CAD build for the part. Positions are in the model's coordinates, mm. Face numbers are marked on the shaded views. A direction names the side the tool comes from. Coordinates: 2 decimals unless noted, no trailing zeros. Loops run counter-clockwise (first coordinate to the right, second up) from the corner with the lowest first, then second, coordinate; pieces in that order, holes last. Notation, with made-up numbers: (70.25, -6) -> (124.25, -6) arc R20 ccw to (124.25, 5) -> close; hole circle Ø1 at (13.5, 64). An arc over 180 degrees is marked (long way). Answer as a JSON object with one key per item and string values. Group by question number.
from build123d import *

# Parameters (mm, degrees)
F0_W     = 33.2
F0_H     = 10.3
F0_R     = 1.75
F1_DEPTH = 1.5
F2_W     = 12.64
F2_H     = 6.3
F3_DEPTH = 4
F4_W     = 4.33
F4_H     = 6.3
F5_DEPTH = 8.4
F6_W     = 5.78
F6_H     = 10.3
F7_DEPTH = 7.6


with BuildPart() as f1:
    # F0 (on Top) → F1 (new body)
    with BuildSketch(Plane.XY):
        with Locations((16.6, -5.15)):
            Rectangle(F0_W, F0_H)
        with Locations((11.11, -5.15)):
            Circle(F0_R, mode=Mode.SUBTRACT)
        with Locations((30.11, -5.15)):
            Circle(F0_R, mode=Mode.SUBTRACT)
    extrude(amount=F1_DEPTH)

    # F2 (on face) → F3 (join)
    with BuildSketch(Plane.XY.offset(1.5)):
        with Locations((20.48, -5.05)):
            Rectangle(F2_W, F2_H)
    extrude(amount=F3_DEPTH)

    # F4 (on face) → F5 (join)
    with BuildSketch(Plane.XY.offset(5.5)):
        with Locations((16.325, -5.05)):
            Rectangle(F4_W, F4_H)
        with Locations((24.635, -5.05)):
            Rectangle(F4_W, F4_H)
    extrude(amount=F5_DEPTH)

    # F6 (on face) → F7 (join)
    with BuildSketch(Plane(origin=(0, 0, 0), x_dir=(1, 0, 0), z_dir=(0, 0, -1))):
        with Locations((3.59, 5.15)):
            Rectangle(F6_W, F6_H)
    extrude(amount=F7_DEPTH)


solid = f1.part
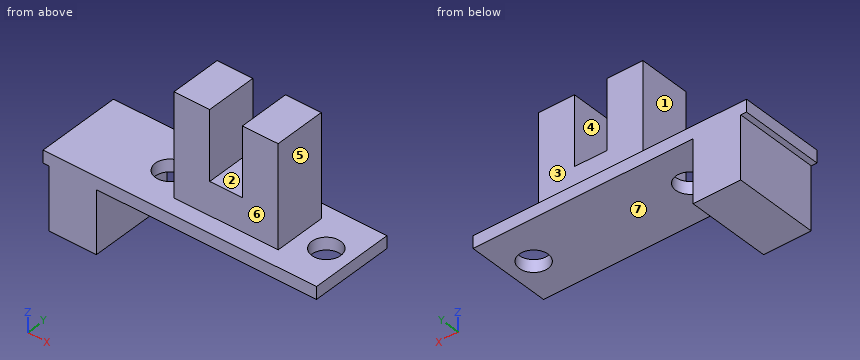
Item 1: Band-saw the part on A-A, the plane z = 8.5. List the corners of the cut face in (x, y), and give its area (3 significant figures).
Item 2: Flat gauge pins, fed straight in: P1, Ø10, axis at x = 19.5, z = 5.5, coming from the -Y side; P2, Ø3, axis at y = -7, z = 11.5, coming from the -X side; P3, Ø4, axis at y = -3.5, z = -4, coming from the -X side; P4, Ø6, axis at y = -6, z = -5, coming from the +X side. Where does each tip first touch, or does it go through?
Item 3: Band-saw the part on C-C, the plane x = 30.11. List the corners of the cut face in (y, z).
Item 4: Drill centre lines: L1, parallel to Y at x = 11.11, z = 0.4; L2, parallel to X at y = -2.5, z = 10; L3, parallel to Z at x = 21, y = -4. Where is each one in solid material? Low to high.
Item 5: Band-saw the part on D-D, the plane x = 21. List the corners of the cut face in (y, z).
Item 6: Pull direction X, two halves, no side cores. Call the marked faces 1, 2 and 3: +X half, -X half, draft (parallel to the pull), parting line (faces both ways), or undercut.
Item 7: 3-axis set-ups, long thin cutter, end or side, ignore diameter. For the marked faces 4, 5, 6 and 7: which of +Z, -Z, +X, -X, +Y, -Y reach the whole face in a straight line?
Item 8: Band-saw the part on B-B, the plane y = -5.15. List the corners of the cut face in (x, z), and give its area (3 significant figures).
Reply:
{
 "1": {"outline": "(14.16, -8.2) -> (18.49, -8.2) -> (18.49, -1.9) -> (14.16, -1.9) -> close; (22.47, -8.2) -> (26.8, -8.2) -> (26.8, -1.9) -> (22.47, -1.9) -> close", "area": "54.6 mm²"},
 "2": {"P1": "y = -10.3", "P2": "x = 14.16", "P3": "x = 0.7", "P4": "x = 6.48"},
 "3": {"outline": "(-10.3, 0) -> (-6.9, 0) -> (-6.9, 1.5) -> (-10.3, 1.5) -> close; (-3.4, 0) -> (0, 0) -> (0, 1.5) -> (-3.4, 1.5) -> close"},
 "4": {"L1": "-10.3 to -6.9, -3.4 to 0", "L2": "14.16 to 18.49, 22.47 to 26.8", "L3": "0 to 5.5"},
 "5": {"outline": "(-10.3, 0) -> (0, 0) -> (0, 1.5) -> (-1.9, 1.5) -> (-1.9, 5.5) -> (-8.2, 5.5) -> (-8.2, 1.5) -> (-10.3, 1.5) -> close"},
 "6": {"face 1": "-X half", "face 2": "undercut", "face 3": "draft"},
 "7": {"face 4": "+Z, +Y, -Y", "face 5": "+Z, +X, +Y, -Y", "face 6": "+Z, +X, -X, -Y", "face 7": "-Z, +X, +Y, -Y"},
 "8": {"outline": "(0, 0) -> (0.7, 0) -> (0.7, -7.6) -> (6.48, -7.6) -> (6.48, 0) -> (9.36, 0) -> (9.36, 1.5) -> (0, 1.5) -> close; (12.86, 0) -> (28.36, 0) -> (28.36, 1.5) -> (26.8, 1.5) -> (26.8, 13.9) -> (22.47, 13.9) -> (22.47, 5.5) -> (18.49, 5.5) -> (18.49, 13.9) -> (14.16, 13.9) -> (14.16, 1.5) -> (12.86, 1.5) -> close; (31.86, 0) -> (33.2, 0) -> (33.2, 1.5) -> (31.86, 1.5) -> close", "area": "207 mm²"}
}
